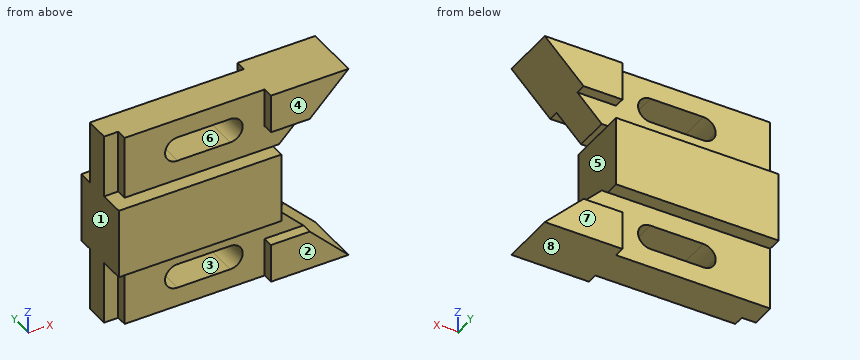
```python
from build123d import *

# Parameters (mm, degrees)
F1_DEPTH  = 104.648
F2_W      = 69.596
F2_H      = 4.826
F3_DEPTH  = 28.575
F2_W_2    = 31.242
F2_H_2    = 1.524
F4_DEPTH  = 150.7
F6_DEPTH  = 28.575
F8_DEPTH  = 26.925
F9_DEPTH  = 4.826
F11_DEPTH = 4.826
F13_DEPTH = 26.925


with BuildPart() as f1:
    # F0 (on Right) → F1 (new body)
    with BuildSketch(Plane.YZ):
        Polygon((0, 28.575), (0, 0), (25.4, 0), (25.4, 28.575), (26.924, 28.575), (26.924, 60.325), (25.4, 60.325), (25.4, 88.9), (0, 88.9), (0, 60.325), (-1.524, 60.325), (-1.524, 28.575), align=None)
    extrude(amount=F1_DEPTH)

    # F2 (on face) → F3 (cut)
    with BuildSketch(Plane.XY.offset(88.9)):
        with Locations((34.798, 22.987)):
            Rectangle(F2_W, F2_H)
        Polygon((0, 4.826), (0, 0), (69.596, 0), (69.596, 4.826), (6.35, 4.826), (6.35, 9.652), (0, 9.652), align=None)
    extrude(amount=-F3_DEPTH, mode=Mode.SUBTRACT)

    # F2 (on face) → F4 (cut)
    with BuildSketch(Plane.XY.offset(88.9)):
        with Locations((89.027, 26.162)):
            Rectangle(F2_W_2, F2_H_2)
        with Locations((89.027, -0.762)):
            Rectangle(F2_W_2, F2_H_2)
    extrude(amount=-F4_DEPTH, mode=Mode.SUBTRACT)

    # F5 (on face) → F6 (cut)
    with BuildSketch(Plane(origin=(0, 0, 0), x_dir=(1, 0, 0), z_dir=(0, 0, -1))):
        Polygon((6.35, -9.652), (6.35, -4.826), (69.596, -4.826), (69.596, 0), (73.406, 0), (73.406, 1.524), (0, 1.524), (0, -9.652), align=None)
        Polygon((69.596, -20.574), (0, -20.574), (0, -26.924), (73.406, -26.924), (73.406, -25.4), (69.596, -25.4), align=None)
    extrude(amount=-F6_DEPTH, mode=Mode.SUBTRACT)

    # F7 (on face) → F8 (cut, through all)
    with BuildSketch(Plane.XZ):
        Polygon((104.648, 44.45), (104.648, 88.9), (87.122, 71.374), (76.073, 60.325), (73.406, 60.325), (73.406, 44.45), align=None)
        Polygon((104.648, 0), (104.648, 44.45), (73.406, 44.45), (73.406, 28.575), (76.073, 28.575), (87.122, 17.526), align=None)
    extrude(amount=-F8_DEPTH, mode=Mode.SUBTRACT)

    # F7 (on face) → F9 (cut)
    with BuildSketch(Plane.XZ):
        Polygon((76.073, 60.325), (87.122, 71.374), (69.596, 71.374), (69.596, 60.325), (73.406, 60.325), align=None)
        Polygon((69.596, 17.526), (87.122, 17.526), (76.073, 28.575), (73.406, 28.575), (69.596, 28.575), align=None)
    extrude(amount=-F9_DEPTH, mode=Mode.SUBTRACT)

    # F10 (on face) → F11 (cut)
    with BuildSketch(Plane(origin=(0, 25.4, 0), x_dir=(-1, 0, 0), z_dir=(0, 1, 0))):
        Polygon((-69.596, 60.325), (-69.596, 71.374), (-87.122, 71.374), (-76.073, 60.325), (-73.406, 60.325), align=None)
        Polygon((-69.596, 17.526), (-69.596, 28.575), (-73.406, 28.575), (-76.073, 28.575), (-87.122, 17.526), align=None)
    extrude(amount=-F11_DEPTH, mode=Mode.SUBTRACT)

    # F12 (on face) → F13 (cut, through all)
    with BuildSketch(Plane.XZ):
        with BuildLine():
            ThreePointArc((30.226, 19.812), (26.2746873067, 18.1753126933), (24.638, 14.224))
            Line((24.638, 14.224), (30.226, 14.224))
            Line((30.226, 14.224), (35.814, 14.224))
            ThreePointArc((35.814, 14.224), (34.1773126933, 18.1753126933), (30.226, 19.812))
        make_face()
        with BuildLine():
            Line((30.226, 14.224), (24.638, 14.224))
            ThreePointArc((24.638, 14.224), (26.2746873067, 10.2726873067), (30.226, 8.636))
            ThreePointArc((30.226, 8.636), (34.1773126933, 10.2726873067), (35.814, 14.224))
            Line((35.814, 14.224), (30.226, 14.224))
        make_face()
        with BuildLine():
            Line((54.102, 19.812), (30.226, 19.812))
            ThreePointArc((30.226, 19.812), (34.1773126933, 18.1753126933), (35.814, 14.224))
            Line((35.814, 14.224), (48.514, 14.224))
            ThreePointArc((48.514, 14.224), (50.1506873067, 18.1753126933), (54.102, 19.812))
        make_face()
        with BuildLine():
            ThreePointArc((35.814, 14.224), (34.1773126933, 10.2726873067), (30.226, 8.636))
            Line((30.226, 8.636), (54.102, 8.636))
            ThreePointArc((54.102, 8.636), (50.1506873067, 10.2726873067), (48.514, 14.224))
            Line((48.514, 14.224), (35.814, 14.224))
        make_face()
        with BuildLine():
            ThreePointArc((59.69, 14.224), (58.0533126933, 18.1753126933), (54.102, 19.812))
            ThreePointArc((54.102, 19.812), (50.1506873067, 18.1753126933), (48.514, 14.224))
            Line((48.514, 14.224), (59.69, 14.224))
        make_face()
        with BuildLine():
            ThreePointArc((48.514, 14.224), (50.1506873067, 10.2726873067), (54.102, 8.636))
            ThreePointArc((54.102, 8.636), (58.0533126933, 10.2726873067), (59.69, 14.224))
            Line((59.69, 14.224), (48.514, 14.224))
        make_face()
        with BuildLine():
            Line((48.514, 74.856311358), (59.69, 74.856311358))
            ThreePointArc((59.69, 74.856311358), (58.0533126933, 78.8076240512), (54.102, 80.444311358))
            ThreePointArc((54.102, 80.444311358), (50.1506873067, 78.8076240512), (48.514, 74.856311358))
        make_face()
        with BuildLine():
            ThreePointArc((54.102, 69.268311358), (58.0533126933, 70.9049986647), (59.69, 74.856311358))
            Line((59.69, 74.856311358), (48.514, 74.856311358))
            ThreePointArc((48.514, 74.856311358), (50.1506873067, 70.9049986647), (54.102, 69.268311358))
        make_face()
        with BuildLine():
            ThreePointArc((48.514, 74.856311358), (50.1506873067, 78.8076240512), (54.102, 80.444311358))
            Line((54.102, 80.444311358), (30.226, 80.444311358))
            ThreePointArc((30.226, 80.444311358), (34.1773126933, 78.8076240512), (35.814, 74.856311358))
            Line((35.814, 74.856311358), (48.514, 74.856311358))
        make_face()
        with BuildLine():
            Line((30.226, 69.268311358), (54.102, 69.268311358))
            ThreePointArc((54.102, 69.268311358), (50.1506873067, 70.9049986647), (48.514, 74.856311358))
            Line((48.514, 74.856311358), (35.814, 74.856311358))
            ThreePointArc((35.814, 74.856311358), (34.1773126933, 70.9049986647), (30.226, 69.268311358))
        make_face()
        with BuildLine():
            ThreePointArc((35.814, 74.856311358), (34.1773126933, 78.8076240512), (30.226, 80.444311358))
            ThreePointArc((30.226, 80.444311358), (26.2746873067, 78.8076240512), (24.638, 74.856311358))
            Line((24.638, 74.856311358), (35.814, 74.856311358))
        make_face()
        with BuildLine():
            ThreePointArc((24.638, 74.856311358), (26.2746873067, 70.9049986647), (30.226, 69.268311358))
            ThreePointArc((30.226, 69.268311358), (34.1773126933, 70.9049986647), (35.814, 74.856311358))
            Line((35.814, 74.856311358), (24.638, 74.856311358))
        make_face()
    extrude(amount=-F13_DEPTH, mode=Mode.SUBTRACT)


solid = f1.part
```
Model file for the job. Use its own axes, mm. Face numbers are marked on the shaded views. A direction names the side the tool comes from. Give positions to 0.01 mm unless a question says otherwise; leave off trailing zeros. Write each loop counter-clockwise with the first axis right and the second up, starting at its lowest first coordinate (ties: lowest second). Pieces come first, ordered by that corner, then holes. Notation, with made-up numbers: (38.25, -1) - (57.25, -1) arc R25 ccw to (57.25, 14) - close; hole circle Ø10 at (-9, 73). An arc over 180 degrees is marked (long way). One line per question, with ' | ' between items. Start each with the question number.
(1) Pin check, flat tips, straight feed: P1, Ø14.5, axis at x = 56.5, z = 71, coming from the +Y side; P2, Ø1.5, axis at y = 17.5, z = 32.5, coming from the +X side; P3, Ø19.5, axis at x = 82, z = 10.5, coming from the +Y side. Stop position of each tip, or through.
(2) Two-plate mould, pull along X, no slides. Class the marked faces 1, 2 and 3: +X half, -X half, draft (parallel to the pull), parting line (faces both ways), or undercut.
(3) 3-axis set-ups, long thin cutter, end or side, ignore diameter. For the marked faces 4, 5, 6, 7 and 8: which of +Z, -Z, +X, -X, +Y, -Y reach the whole face in a straight line?
(4) Slice it at C-C on y = 8.5. Write the cut outline in (x, z) (3 decimals), plus the area to 3 significant figures.
(5) Wall check: line 1 along Z through (x, y) = (38, 11.25); line 2 along Z through (x, y) = (77, 2); line 3 along Z through (x, y) = (4, 21.25) (3 decimals). Give the ranges that are in metal, low to high. Write a range as from..to.
(6) Slice it at A-A on y = 1.5. Write the cut outline in (x, z) (3 decimals).
(7) Slice it at D-D on z = 78.5. Write the cut outline in (x, y), plus the area to 3 significant figures.
(8) Slice it at B-B on x = 36.5. Write the cut outline in (y, z) (3 decimals), plus the area to 3 significant figures.
Results below:
1) P1: y = 20.57 | P2: x = 73.41 | P3: y = 25.4
2) face 1: -X half | face 2: draft | face 3: undercut
3) face 4: +Z, +X, -X, -Y | face 5: +X, +Y, -Y | face 6: +Y, -Y | face 7: -Z, +X, -X, +Y | face 8: -Z, +X, -X, +Y, -Y
4) outline: (0, 28.575) - (6.35, 28.575) - (6.35, 0) - (104.648, 0) - (76.073, 28.575) - (73.406, 28.575) - (73.406, 60.325) - (76.073, 60.325) - (104.648, 88.9) - (6.35, 88.9) - (6.35, 60.325) - (0, 60.325) - close; hole (30.226, 8.636) - (54.102, 8.636) arc R5.588 ccw to (54.102, 19.812) - (30.226, 19.812) arc R5.588 ccw to start; hole (30.226, 69.268) - (54.102, 69.268) arc R5.588 ccw to (54.102, 80.444) - (30.226, 80.444) arc R5.588 ccw to start | area: 6,400 mm^2
5) line 1: 0..8.64, 19.81..69.27, 80.44..88.9 | line 2: 0..17.53, 71.37..88.9 | line 3: 28.575..60.325
6) outline: (0, 28.575) - (73.406, 28.575) - (73.406, 60.325) - (0, 60.325) - close; (69.596, 0) - (104.648, 0) - (87.122, 17.526) - (69.596, 17.526) - close; (69.596, 71.374) - (87.122, 71.374) - (104.648, 88.9) - (69.596, 88.9) - close
7) outline: (0, 9.65) - (6.35, 9.65) - (6.35, 4.83) - (25.99, 4.83) - (25.99, 20.57) - (0, 20.57) - close; (58.34, 4.83) - (69.6, 4.83) - (69.6, 0) - (94.25, 0) - (94.25, 25.4) - (69.6, 25.4) - (69.6, 20.57) - (58.34, 20.57) - close | area: 1,180 mm^2
8) outline: (-1.524, 28.575) - (4.826, 28.575) - (4.826, 19.812) - (20.574, 19.812) - (20.574, 28.575) - (26.924, 28.575) - (26.924, 60.325) - (20.574, 60.325) - (20.574, 69.268) - (4.826, 69.268) - (4.826, 60.325) - (-1.524, 60.325) - close; (4.826, 0) - (20.574, 0) - (20.574, 8.636) - (4.826, 8.636) - close; (4.826, 80.444) - (20.574, 80.444) - (20.574, 88.9) - (4.826, 88.9) - close | area: 1,450 mm^2
